Input: part model. Units: mm. Frame: model coordinates. Round coordinates to 2 decimals unless told otherwise and drop trailing zeros. Order: outer loops, then holes, each group sorted by start corner. A loop starts at its lowest first (then second) coordinate and runs counter-clockwise, first axis right, second up. Notation, with made-up numbers: (88.5, 29.5) -> (111.5, 29.5) arc R28 ccw to (111.5, 68.5) -> close; hole circle Ø6 at (51, -25). An arc over 180 degrees is marked (long way). Use a Markdown table: item, result.
from build123d import *

# Parameters (mm, degrees)
F0_W     = 10
F0_H     = 10
F1_DEPTH = 350
F3_DEPTH = 25
F5_DEPTH = 10.001


with BuildPart() as f1:
    # F0 (on Front) → F1 (new body)
    with BuildSketch(Plane.XZ):
        with Locations((5, 5)):
            Rectangle(F0_W, F0_H)
    extrude(amount=F1_DEPTH)

    # F2 (on face) → F3 (cut)
    with BuildSketch(Plane(origin=(0, 0, 0), x_dir=(0, -1, 0), z_dir=(-1, 0, 0))):
        Polygon((62.5, 7.5), (65, 10), (60, 10), align=None)
        Polygon((87.5, 7.5), (90, 10), (85, 10), align=None)
        Polygon((112.5, 7.5), (115, 10), (110, 10), align=None)
        Polygon((137.5, 7.5), (140, 10), (135, 10), align=None)
        Polygon((162.5, 7.5), (165, 10), (160, 10), align=None)
        Polygon((187.5, 7.5), (190, 10), (185, 10), align=None)
        Polygon((212.5, 7.5), (215, 10), (210, 10), align=None)
        Polygon((237.5, 7.5), (240, 10), (235, 10), align=None)
        Polygon((262.5, 7.5), (265, 10), (260, 10), align=None)
        Polygon((287.5, 7.5), (290, 10), (285, 10), align=None)
    extrude(amount=-F3_DEPTH, mode=Mode.SUBTRACT)

    # F4 (on face) → F5 (cut, through all)
    with BuildSketch(Plane.XY.offset(10)):
        with BuildLine():
            Line((8, -45), (8, -35))
            ThreePointArc((8, -35), (5, -32), (2, -35))
            Line((2, -35), (2, -45))
            ThreePointArc((2, -45), (5, -48), (8, -45))
        make_face()
        with BuildLine():
            Line((7.916715, -315), (7.916715, -305))
            ThreePointArc((7.916715, -305), (4.916715, -302), (1.916715, -305))
            Line((1.916715, -305), (1.916715, -315))
            ThreePointArc((1.916715, -315), (4.916715, -318), (7.916715, -315))
        make_face()
    extrude(amount=-F5_DEPTH, mode=Mode.SUBTRACT)


solid = f1.part
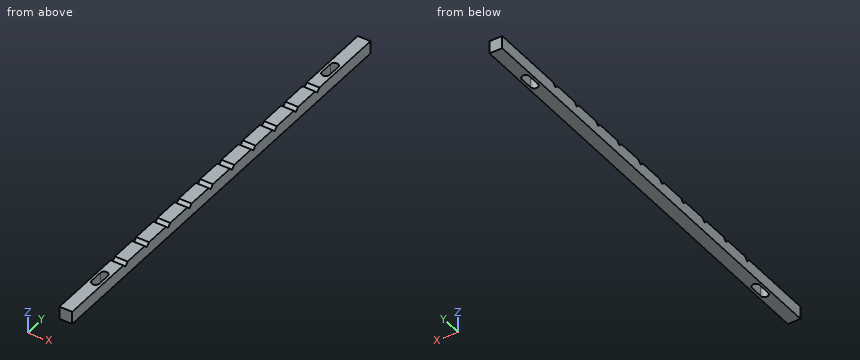
1) Cut plane A-A on z = 3.75. Return loops of the section in (x, y), and give its area (3 significant figures).
Results found:
| item | result |
|---|---|
| outline | (0, -350) -> (10, -350) -> (10, 0) -> (0, 0) -> close; hole (1.92, -315) arc R3 ccw to (7.92, -315) -> (7.92, -305) arc R3 ccw to (1.92, -305) -> close; hole (2, -45) arc R3 ccw to (8, -45) -> (8, -35) arc R3 ccw to (2, -35) -> close |
| area | 3,320 mm² |
2) Line query: L1, parallel to Y at x = 5.25, z = 7; L2, parallel to X at y = -305, z = 4.25; L3, parallel to Y at x = 5.5, z = 4. Output: solid intervals per line, ascending. Write a range as [from, to].
Results found:
| item | result |
|---|---|
| L1 | y = [-350, -317.98], [-302.02, -47.99], [-32.01, 0] |
| L2 | x = [0, 1.92], [7.92, 10] |
| L3 | y = [-350, -317.94], [-302.06, -47.96], [-32.04, 0] |
3) Cut plane B-B on x = 5. Count the separate pieces of the cut face and the enclosed holes in it, and give its area (3 significant figures).
Results found:
| item | result |
|---|---|
| separate pieces | 3 |
| enclosed holes | 0 |
| area | 3,120 mm² |
4) Pin query (flat end, axial travel): pin 1 Ø2 at (x, y) = (3.5, -288.5) entering from +Z; pin 2 Ø1.5 at (x, y) = (3, -162.5) entering from +Z. Return the tip coordinate at first contact, or that it passes through.
Results found:
| item | result |
|---|---|
| pin 1 | stops at z = 9.5 |
| pin 2 | stops at z = 8.25 |
